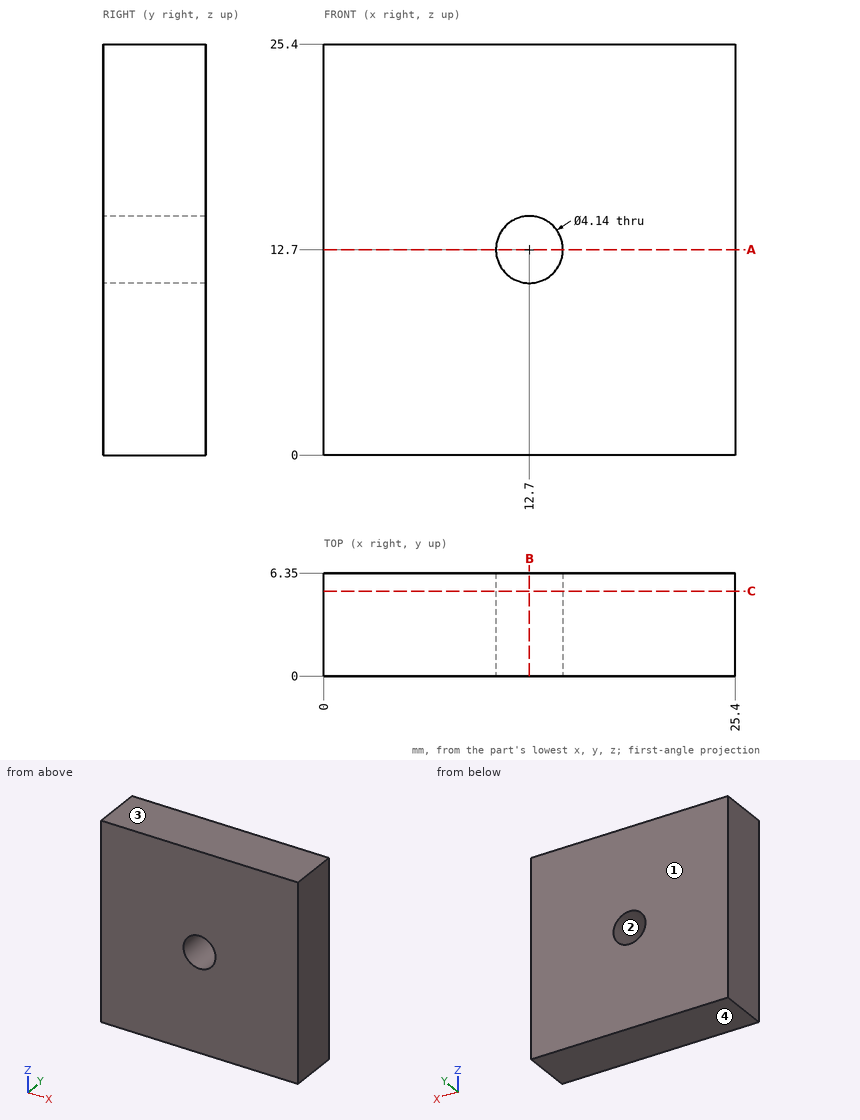
Here's the drawing with two shaded views (mm, measured from the low corner). I have some questions. Give positions to 0.01 mm unless a question says otherwise; leave off trailing zeros. Write each loop counter-clockwise with the first axis right and the second up, starting at its lowest first coordinate (ties: lowest second). Pieces come first, ordered by that corner, then holes. Notation, with made-up numbers: (14, 10.25) -> (70, 10.25) arc R17 cw to (70, 38.25) -> close; hole circle Ø9 at (2.5, 61.25). An arc over 180 degrees is marked (long way). Use one line per item in the form item = value. Start each with the question number.
1. Thinking about a two-plate mould opening in Z: for the marked faces 1, 2, 3 and 4, which applies, +Z half, -Z half, draft (parallel to the pull), parting line (faces both ways), or undercut?
2. Imagine slicing it at A-A on z = 12.7. List the corners of the cut face in (x, y) for me, plus the area to 3 significant figures.
3. If I drill on L1, parallel to Z at x = 12.7, y = 2; L2, parallel to X at y = 1.75, z = 11.25, over which ranges is the centre line in solid material (lowest first)?
4. Imagine slicing it at C-C on y = 5.25. List the corners of the cut face in (x, z) for me.
5. Imagine slicing it at B-B on x = 12.7. List the corners of the cut face in (y, z) for me.
Entries:
q1.face_1 = draft
q1.face_2 = undercut
q1.face_3 = +Z half
q1.face_4 = -Z half
q2.outline = (0, 0) -> (10.63, 0) -> (10.63, 6.35) -> (0, 6.35) -> close; (14.77, 0) -> (25.4, 0) -> (25.4, 6.35) -> (14.77, 6.35) -> close
q2.area = 135 mm²
q3.L1 = 0 to 10.63, 14.77 to 25.4
q3.L2 = 0 to 11.22, 14.18 to 25.4
q4.outline = (0, 0) -> (25.4, 0) -> (25.4, 25.4) -> (0, 25.4) -> close; hole circle Ø4.14 at (12.7, 12.7)
q5.outline = (0, 0) -> (6.35, 0) -> (6.35, 10.63) -> (0, 10.63) -> close; (0, 14.77) -> (6.35, 14.77) -> (6.35, 25.4) -> (0, 25.4) -> close
